from build123d import *

# Parameters (mm, degrees)
F0_W     = 230
F0_H     = 20
F1_DEPTH = 2.5
F3_D     = 3.3
F4_SIZE2 = 4
F4_SIZE  = 1
F6_D     = 8
F6_DEPTH = 0.2
F6_TIP   = 2.4034424761


with BuildPart() as f1:
    # F0 (on Top) → F1 (new body)
    with BuildSketch(Plane.XY):
        Rectangle(F0_W, F0_H)
    extrude(amount=F1_DEPTH)

    # F3 (through all)
    with Locations(Plane.XY.offset(2.5)):
        with Locations((-105, -5), (-70, -5), (-35, -5), (0, -5), (35, -5), (105, -5), (70, -5)):
            Hole(F3_D / 2)

    # F4
    f4_edges = [f1.edges().sort_by_distance(p)[0] for p in [
        (0, 10, 0),
    ]]
    f4_side = f1.faces().sort_by_distance((0, 10, 1.25))[0]
    chamfer(f4_edges, length=F4_SIZE, length2=F4_SIZE2, reference=f4_side)

    # F6
    with Locations(Plane.XY.offset(2.5)):
        with Locations((-105, -5), (-70, -5), (-35, -5), (0, -5), (105, -5), (70, -5), (35, -5)):
            Hole(F6_D / 2, depth=F6_DEPTH)
            with Locations((0, 0, -(F6_DEPTH + F6_TIP / 2))):  # 118° drill point
                Cone(0, F6_D / 2, F6_TIP, mode=Mode.SUBTRACT)


solid = f1.part
Here's how the part is built. I have some questions about the finished solid (model axes, mm). Coordinates: 2 decimals unless noted, no trailing zeros. Loops run counter-clockwise (first coordinate to the right, second up) from the corner with the lowest first, then second, coordinate; pieces in that order, holes last.
1. Imagine slicing it at A-A, the plane z = 1.7. Please give me the cut outline in (x, y).
2. I need wall thicknesses on L1, parallel to Y at x = -35, z = 2.35; L2, parallel to Z at x = -67, y = 7.5 (3 decimals); L3, parallel to Z at x = 31.5, y = -3.5. Which ranges of each line are inside material? Lowest first, please.
3. For P1, Ø6.5, axis at x = 35, y = -5, coming from the +Z side; P2, Ø3, axis at x = 35, y = -5, coming from the -Z side; P3, Ø4, axis at x = 69.5, y = -4.5, coming from the +Z side; P4, Ø7, axis at x = -105, y = -5, coming from the +Z side, each with a flat end and sliding along its axis, tell me the tip position at first contact or that it passes through.
4. Imagine slicing it at B-B, the plane x = 45. Please give me the cut outline in (y, z).
5. If we mould it in two halves opening along X, with no side actions, what happens to faces 1 (the flat face through (-2, 0, 2.5)), 2 (the conical face through (-106.426, -6.093, 0.976))? For each: pulls with the +X half, pulls with the -X half, needs draft (parallel to the pull), parting line crosses it, or undercut.
Taken from the geometry:
1. outline: (-115, -10) - (115, -10) - (115, 10) - (-115, 10) - close; hole circle Ø6 at (-105, -5); hole circle Ø6 at (-70, -5); hole circle Ø6 at (-35, -5); hole circle Ø6 at (0, -5); hole circle Ø6 at (35, -5); hole circle Ø6 at (70, -5); hole circle Ø6 at (105, -5)
2. L1: y = -10 to -9, -1 to 10
2. L2: z = 0.375 to 2.5
2. L3: z = 0 to 2.18
3. P1: stops at z = 1.85
3. P2: passes through
3. P3: stops at z = 1.52
3. P4: stops at z = 2
4. outline: (-10, 0) - (6, 0) - (10, 1) - (10, 2.5) - (-10, 2.5) - close
5. face 1: needs draft
5. face 2: undercut
